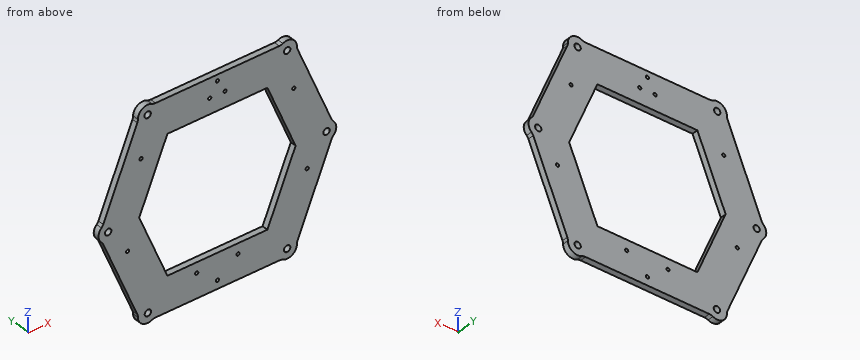
```python
from build123d import *

# Parameters (mm, degrees)
BOSS_EXTRUDE2_DEPTH             = 4.7752
CUT_EXTRUDE1_DEPTH              = 124.57218077
CUT_EXTRUDE1_DEPTH_BACK         = 124.57218077
F_2_5MM_DOWEL_HOLE1_D           = 2.5
F_2_5MM_DOWEL_HOLE1_CSINK_D     = 2.55
F_2_5MM_DOWEL_HOLE1_CSINK_ANGLE = 90
SKETCH7_R                       = 7.62
BOSS_EXTRUDE3_DEPTH             = 4.7752
FILLET1_R                       = 6.35
F_5_0MM_DOWEL_HOLE1_D           = 5
F_5_0MM_DOWEL_HOLE1_CSINK_D     = 5.05
F_5_0MM_DOWEL_HOLE1_CSINK_ANGLE = 90


with BuildPart() as part:
    # Sketch1 → Boss-Extrude2 (new body)
    with BuildSketch(Plane(origin=(0, 0, 0), x_dir=(1, 0, 0), z_dir=(0, 1, 0))):
        Polygon((-59.461458223, 81.205013652), (-93.021648464, 0), (-59.461458223, -81.205013652), (59.461458223, -81.205013652), (93.021648464, 0), (59.461458223, 81.205013652), align=None)
    extrude(amount=BOSS_EXTRUDE2_DEPTH)

    # Sketch4 → Cut-Extrude1 (cut, two sides: drawn at the far end of the back side and taken through both)
    with BuildSketch(Plane.XZ.offset(-CUT_EXTRUDE1_DEPTH_BACK)):
        Polygon((-39.361989183, 53.755675768), (-61.577990685, 0), (-39.361989183, -53.755675768), (39.361989183, -53.755675768), (61.577990685, 0), (39.361989183, 53.755675768), align=None)
    extrude(amount=CUT_EXTRUDE1_DEPTH + CUT_EXTRUDE1_DEPTH_BACK, mode=Mode.SUBTRACT)

    # Ø2.5mm Dowel Hole1 (through all)
    with Locations(Plane(origin=(-6.03758, 0, 65.965013652), x_dir=(0, 0, -1), z_dir=(0, -1, 0))):
        with Locations((0, 0), (0, 12.07516), (127.889, -10.25652), (127.889, 22.33168), (140.589, 6.03758), (-10.414, 6.03758), (21.888921631, -54.068737531), (87.314572085, -64.692973675), (87.314572085, 76.768133675), (21.888921631, 66.143897531)):
            CounterSinkHole(F_2_5MM_DOWEL_HOLE1_D / 2, F_2_5MM_DOWEL_HOLE1_CSINK_D / 2, counter_sink_angle=F_2_5MM_DOWEL_HOLE1_CSINK_ANGLE)

    # Sketch7 → Boss-Extrude3 (add)
    with BuildSketch(Plane.XZ):
        with Locations((-54.959644352, 75.057)):
            Circle(SKETCH7_R)
        with Locations((54.959644352, 75.057)):
            Circle(SKETCH7_R)
        with Locations((85.979, 0)):
            Circle(SKETCH7_R)
        with Locations((54.959644352, -75.057)):
            Circle(SKETCH7_R)
        with Locations((-54.959644352, -75.057)):
            Circle(SKETCH7_R)
        with Locations((-85.979, 0)):
            Circle(SKETCH7_R)
    extrude(amount=-BOSS_EXTRUDE3_DEPTH)

    # Fillet1
    fillet1_edges = [part.edges().sort_by_distance(p)[0] for p in [
        (-62.488338925, 2.3876, 73.880922611),
        (-50.45783048, 2.3876, 81.205013652),
        (50.45783048, 2.3876, 81.205013652),
        (62.488338925, 2.3876, 73.880922611),
        (90.480813872, 2.3876, 6.148013652),
        (90.480813872, 2.3876, -6.148013652),
        (50.45783048, 2.3876, -81.205013652),
        (62.488338925, 2.3876, -73.880922611),
        (-50.45783048, 2.3876, -81.205013652),
        (-62.488338925, 2.3876, -73.880922611),
        (-90.480813872, 2.3876, -6.148013652),
        (-90.480813872, 2.3876, 6.148013652),
    ]]
    fillet(fillet1_edges, radius=FILLET1_R)

    # Ø5.0mm Dowel Hole1 (through all)
    with Locations(Plane(origin=(-54.959644352, 0, 75.057), x_dir=(0, 0, -1), z_dir=(0, -1, 0))):
        with Locations((0, 0), (150.062149462, 109.88132173), (150.114, 0.244119934), (75.057, -31.019355648), (75.057, 140.938644352), (0, 109.919288704)):
            CounterSinkHole(F_5_0MM_DOWEL_HOLE1_D / 2, F_5_0MM_DOWEL_HOLE1_CSINK_D / 2, counter_sink_angle=F_5_0MM_DOWEL_HOLE1_CSINK_ANGLE)


solid = part.part
```
Input: part model. Units: mm. Frame: model coordinates. Give positions to 0.01 mm unless a question says otherwise; leave off trailing zeros. Order: outer loops, then holes, each group sorted by start corner. A loop starts at its lowest first (then second) coordinate and runs counter-clockwise, first axis right, second up. Notation, with made-up numbers: (47, 21) - (89, 21) arc R9 cw to (89, 37) - close; hole circle Ø3 at (42, 57.5). An arc over 180 degrees is marked (long way). Use a Markdown table: item, result.
(1) Section query A-A (x = -33.5). Output: boundary loops of the cut face in (y, z), then the cut area to 3 significant figures.
Computed values:
| item | result |
|---|---|
| outline | (0, -81.21) - (4.78, -81.21) - (4.78, -53.76) - (0, -53.76) - close; (0, 53.76) - (4.78, 53.76) - (4.78, 81.21) - (0, 81.21) - close |
| area | 262 mm2 |
(2) Line query: line 1 (Z direction, x = -24, y = 4); line 2 (X direction, y = 0.2, z = -74.5); line 3 (X direction, y = 2.85, z = -76). Output: solid intervals per line, ascending. Write a range as from..to.
Computed values:
| item | result |
|---|---|
| line 1 | z = -81.21..-53.76, 53.76..81.21 |
| line 2 | x = -62.59..-57.15, -52.28..-1.24, 1.24..52.47, 57.37..62.59 |
| line 3 | x = -62.52..-57.03, -52.4..52.63, 57.22..62.52 |
(3) Section query B-B (z = -36). Output: boundary loops of the cut face in (x, y), then the cut area to 3 significant figures.
Computed values:
| item | result |
|---|---|
| outline | (-78.14, 0) - (-46.7, 0) - (-46.7, 4.78) - (-78.14, 4.78) - close; (46.7, 0) - (78.14, 0) - (78.14, 4.78) - (46.7, 4.78) - close |
| area | 300 mm2 |
(4) Pin query (flat end, axial travel): pin 1 (1.5 mm diameter, centred on x = -70.73, z = -21.35, fed in from +Y); pin 2 (1 mm diameter, centred on y = 1.5, z = -11, fed in from -X); pin 3 (1.5 mm diameter, centred on x = -49.5, y = 3, fed in from +Z); pin 4 (1.5 mm diameter, centred on x = -35.5, y = 3.5, fed in from +Z) (3 decimals). Return the tip coordinate at first contact, or that it passes through.
Computed values:
| item | result |
|---|---|
| pin 1 | passes through |
| pin 2 | stops at x = -88.68 |
| pin 3 | stops at z = 81.39 |
| pin 4 | stops at z = 81.205 |
(5) Section query C-C (y = 2.65). State how many separate pieces and enclosed holes the cut face has, then the cut area to 3 significant figures.
Computed values:
| item | result |
|---|---|
| separate pieces | 1 |
| enclosed holes | 17 |
| area | 13,800 mm2 |
